Geometry check sheet. Reference: the model listing, model coordinates, mm. A direction names the side the tool comes from. Round coordinates to 2 decimals unless told otherwise and drop trailing zeros. Order: outer loops, then holes, each group sorted by start corner. A loop starts at its lowest first (then second) coordinate and runs counter-clockwise, first axis right, second up. Notation, with made-up numbers: (45, -2.75) - (81, -2.75) arc R18 ccw to (81, 13.25) - close; hole circle Ø8 at (-30, 49). An arc over 180 degrees is marked (long way). Answer as CSV lines item,"result". Start each with the question number.
```python
from build123d import *

# Parameters (mm, degrees)
SKIZZE1_W                                            = 65
SKIZZE1_H                                            = 34
SKIZZE1_R                                            = 9
SKIZZE1_R_2                                          = 4
AUFSATZ_LINEAR_AUSTRAGEN1_DEPTH                      = 3
SCHNITT_LINEAR_START                                 = 3
SKIZZE1_3_R                                          = 10.5
SCHNITT_LINEAR_AUSTRAGEN1_DEPTH                      = 5
SKIZZE1_4_R                                          = 5
SCHNITT_LINEAR_AUSTRAGEN2_DEPTH                      = 3
SCHNITT_LINEAR_AUSTRAGEN4_DEPTH                      = 7
SCHNITT_LINEAR_AUSTRAGEN5_DEPTH                      = 3
VERRUNDUNG1_R                                        = 3
M3_GEWINDEBOHRUNG1_D                                 = 2.5
M3_GEWINDEBOHRUNG1_DEPTH                             = 7
M3_GEWINDEBOHRUNG1_TIP                               = 0.751075774
M3_GEWINDEBOHRUNG2_D                                 = 2.5
M3_GEWINDEBOHRUNG2_DEPTH                             = 7.5
M3_GEWINDEBOHRUNG2_TIP                               = 0.751075774
SKIZZE6_3_OUTSIDE_W                                  = 81.72
SKIZZE6_3_OUTSIDE_H                                  = 50.72
SKIZZE6_3_OUTSIDE_W_2                                = 32.5
SKIZZE6_3_OUTSIDE_H_2                                = 34
NUR_ANTRIEB_DEPTH                                    = 7
VERRUNDUNG3_R                                        = 3
SKIZZE7_R                                            = 5
SCHNITT_LINEAR_AUSTRAGEN3_DEPTH                      = 2.5
STIRNSENKUNG_F_R_M2_5_ZYLINDERSCHRAUBE_M_D           = 2.7
STIRNSENKUNG_F_R_M2_5_ZYLINDERSCHRAUBE_M_CBORE_D     = 5.5
STIRNSENKUNG_F_R_M2_5_ZYLINDERSCHRAUBE_M_CBORE_DEPTH = 1.8


with BuildPart() as part:
    # Skizze1 → Aufsatz-Linear austragen1 (new body, symmetric)
    with BuildSketch(Plane.XY):
        with Locations((0, 1.5)):
            Rectangle(SKIZZE1_W, SKIZZE1_H)
        with Locations((20.5, 0)):
            Circle(SKIZZE1_R, mode=Mode.SUBTRACT)
        with Locations((-22.5, -3)):
            Circle(SKIZZE1_R_2, mode=Mode.SUBTRACT)
    extrude(amount=AUFSATZ_LINEAR_AUSTRAGEN1_DEPTH, both=True)

    # Skizze1<3> → Schnitt-Linear austragen1 (cut)
    with BuildSketch(Plane.XY.offset(SCHNITT_LINEAR_START)):
        with Locations((20.5, 0)):
            Circle(SKIZZE1_3_R)
    extrude(amount=-SCHNITT_LINEAR_AUSTRAGEN1_DEPTH, mode=Mode.SUBTRACT)

    # Skizze1<4> → Schnitt-Linear austragen2 (cut)
    with BuildSketch(Plane.XY.offset(SCHNITT_LINEAR_START)):
        with Locations((-22.5, -3)):
            Circle(SKIZZE1_4_R)
    extrude(amount=-SCHNITT_LINEAR_AUSTRAGEN2_DEPTH, mode=Mode.SUBTRACT)

    # Skizze11 → Schnitt-Linear austragen4 (cut, through all)
    with BuildSketch(Plane(origin=(0, 0, -3), x_dir=(-1, 0, 0), z_dir=(0, 0, -1))):
        with BuildLine():
            Line((9.5, 13.5), (9.5, -10.5))
            ThreePointArc((9.5, -10.5), (7.5, -12.5), (5.5, -10.5))
            Line((5.5, -10.5), (5.5, 13.5))
            ThreePointArc((5.5, 13.5), (7.5, 15.5), (9.5, 13.5))
        make_face()
    extrude(amount=-SCHNITT_LINEAR_AUSTRAGEN4_DEPTH, mode=Mode.SUBTRACT)

    # Skizze11<4> → Schnitt-Linear austragen5 (cut)
    with BuildSketch(Plane(origin=(0, 0, -3), x_dir=(-1, 0, 0), z_dir=(0, 0, -1))):
        with BuildLine():
            Line((11, 13.5), (11, -10.5))
            ThreePointArc((11, -10.5), (7.5, -14), (4, -10.5))
            Line((4, -10.5), (4, 13.5))
            ThreePointArc((4, 13.5), (7.5, 17), (11, 13.5))
        make_face()
    extrude(amount=-SCHNITT_LINEAR_AUSTRAGEN5_DEPTH, mode=Mode.SUBTRACT)

    # Verrundung1
    verrundung1_edges = [part.edges().sort_by_distance(p)[0] for p in [
        (-32.5, 18.5, 0),
        (32.5, 18.5, 0),
    ]]
    fillet(verrundung1_edges, radius=VERRUNDUNG1_R)

    # M3 Gewindebohrung1
    with Locations(Plane(origin=(-30, -15.5, -6.25), x_dir=(-1, 0, 0), z_dir=(0, -1, 0))):
        with Locations((-56.5, -6.75), (-1.5, -6.75), (-44.5, -6.75), (-13.5, -6.75)):
            Hole(M3_GEWINDEBOHRUNG1_D / 2, depth=M3_GEWINDEBOHRUNG1_DEPTH)
            with Locations((0, 0, -(M3_GEWINDEBOHRUNG1_DEPTH + M3_GEWINDEBOHRUNG1_TIP / 2))):  # 118° drill point
                Cone(0, M3_GEWINDEBOHRUNG1_D / 2, M3_GEWINDEBOHRUNG1_TIP, mode=Mode.SUBTRACT)

    # M3 Gewindebohrung2
    with Locations(Plane(origin=(0, 18.5, 0), x_dir=(1, 0, 0), z_dir=(0, 1, 0))):
        with Locations((20.5, 0)):
            Hole(M3_GEWINDEBOHRUNG2_D / 2, depth=M3_GEWINDEBOHRUNG2_DEPTH)
            with Locations((0, 0, -(M3_GEWINDEBOHRUNG2_DEPTH + M3_GEWINDEBOHRUNG2_TIP / 2))):  # 118° drill point
                Cone(0, M3_GEWINDEBOHRUNG2_D / 2, M3_GEWINDEBOHRUNG2_TIP, mode=Mode.SUBTRACT)


with BuildPart() as body_2:
    # Spiegeln1: mirrored copy
    add(part.part.mirror(Plane.XY.offset(3)))

    # Skizze6<3> outside → Nur Antrieb (cut, through all)
    with BuildSketch(Plane(origin=(0, 0, 3), x_dir=(-1, 0, 0), z_dir=(0, 0, -1))):
        with Locations((0, 1.5)):
            Rectangle(SKIZZE6_3_OUTSIDE_W, SKIZZE6_3_OUTSIDE_H)
        with Locations((16.25, 1.5)):
            Rectangle(SKIZZE6_3_OUTSIDE_W_2, SKIZZE6_3_OUTSIDE_H_2, mode=Mode.SUBTRACT)
    extrude(amount=-NUR_ANTRIEB_DEPTH, mode=Mode.SUBTRACT)

    # Verrundung3
    verrundung3_edges = [body_2.edges().sort_by_distance(p)[0] for p in [
        (0, 18.5, 6),
    ]]
    fillet(verrundung3_edges, radius=VERRUNDUNG3_R)

    # Skizze7 → Schnitt-Linear austragen3 (cut)
    with BuildSketch(Plane(origin=(0, 0, 9), x_dir=(-1, 0, 0), z_dir=(0, 0, -1))):
        with Locations((22.5, -3)):
            Circle(SKIZZE7_R)
    extrude(amount=SCHNITT_LINEAR_AUSTRAGEN3_DEPTH, mode=Mode.SUBTRACT)

    # Stirnsenkung für  M2.5 Zylinderschraube mit Schlitz/Kreuzschlitz1 (through all)
    with Locations(Plane(origin=(6.813962519, -2.610238453, 3), x_dir=(1, 0, 0), z_dir=(0, 0, -1))):
        with Locations((-29.313962519, -7.610238453), (-29.313962519, 8.389761547)):
            CounterBoreHole(STIRNSENKUNG_F_R_M2_5_ZYLINDERSCHRAUBE_M_D / 2, STIRNSENKUNG_F_R_M2_5_ZYLINDERSCHRAUBE_M_CBORE_D / 2, STIRNSENKUNG_F_R_M2_5_ZYLINDERSCHRAUBE_M_CBORE_DEPTH)


solid = body_2.part
```
1. Section check A-A on y = 11. Record the boundary of the cut face in (x, z).
2. Section check B-B on x = -22.5. Count the separate pieces of the cut face and the enclosed holes in it, plus the area to 3 significant figures.
3. Access from +Z, -Z, +X, -X, +Y, -Y to the whole of each face (thin tool, end or side, straight path). Record for faces 1 (the face through (-21, 1, 6)), 2 (the face through (-7.4, 17, 7.5)), 3 (the face through (-9.5, 2, 5)).
4. Thickness scan on probe 1 along Y at (x, z) = (-22.5, 3.9); probe 2 along X at (y, z) = (-12.75, 5.5); probe 3 along X at (y, z) = (5, 8). Record the ranges inside material, lowest first.
5. Draft check along X on faces 4 (the face through (-31.64, 17.6, 6.04)), 5 (the face through (-16, -15.5, 7)), 6 (the face through (-23.226, -12.138, 6.929)). Enter one of: released by +X, released by -X, zero draft, split by the parting line, or undercut.
6. Go/stop test with a flat-tipped pin: pin 1 Ø6 at (x, y) = (-22.5, -3) entering from -Z. Record where the tip stops, or that it passes through.
7. Section check C-C on z = 7.2. Record the boundary of the cut face in (x, y), plus the area to 3 significant figures.
8. Section check D-D on y = 5. Record the boundary of the cut face in (x, z).
Numbers:
1,outline,"(-32.5, 3) - (-9.5, 3) - (-9.5, 6) - (-11, 6) - (-11, 9) - (-32.5, 9) - close; (-5.5, 3) - (0, 3) - (0, 9) - (-4, 9) - (-4, 6) - (-5.5, 6) - close"
2,separate pieces,"4"
2,enclosed holes,"0"
2,area,"103 mm2"
3,face 1,"-Z"
3,face 2,"+Z"
3,face 3,"+Z, -Z"
4,probe 1,"y = -15.5 to -13.75, -8.25 to -8, 2 to 2.25, 7.75 to 18.5"
4,probe 2,"x = -32.5 to -29.75, -27.25 to -17.75, -15.25 to 0"
4,probe 3,"x = -32.5 to -23.85, -21.15 to -11, -4 to 0"
5,face 4,"released by -X"
5,face 5,"zero draft"
5,face 6,"undercut"
6,pin 1,"passes through"
7,outline,"(-32.5, -15.5) - (0, -15.5) - (0, 15.5) arc R3 ccw to (-3, 18.5) - (-29.5, 18.5) arc R3 ccw to (-32.5, 15.5) - close; hole circle Ø10 at (-22.5, -3); hole circle Ø2.7 at (-22.5, -11); hole circle Ø2.7 at (-22.5, 5); hole (-11, -10.5) arc R3.5 ccw to (-4, -10.5) - (-4, 13.5) arc R3.5 ccw to (-11, 13.5) - close"
7,area,"805 mm2"
8,outline,"(-32.5, 3) - (-25.25, 3) - (-25.25, 4.8) - (-23.85, 4.8) - (-23.85, 9) - (-32.5, 9) - close; (-21.15, 4.8) - (-19.75, 4.8) - (-19.75, 3) - (-9.5, 3) - (-9.5, 6) - (-11, 6) - (-11, 9) - (-21.15, 9) - close; (-5.5, 3) - (0, 3) - (0, 9) - (-4, 9) - (-4, 6) - (-5.5, 6) - close"
